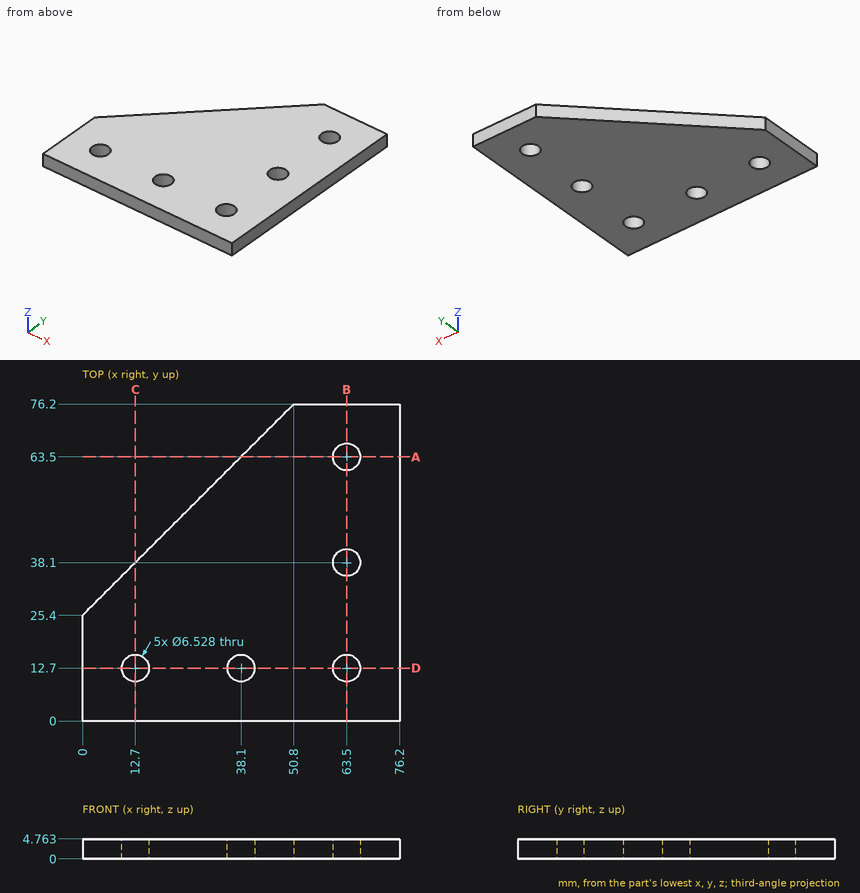
Job drawing, mm, ordinate dimensions from the low corner. One solid piece. Give positions to 0.01 mm unless a question says otherwise; leave off trailing zeros. Write each loop counter-clockwise with the first axis right and the second up, starting at its lowest first coordinate (ties: lowest second). Pieces come first, ordered by that corner, then holes. Notation, with made-up numbers: (89.5, 71.25) - (121.5, 71.25) arc R24 cw to (121.5, 103.25) - close; hole circle Ø5 at (28.25, -1.75). An arc over 180 degrees is marked (long way). Use one line per item in the form item = value. Start each with the question number.
1. Drop flat-ended pins along their axis: pin 1 Ø4 at (x, y) = (38.1, 12.7) entering from +Z; pin 2 Ø1 at (x, z) = (17, 2) entering from +Y. Give the stop position or say it passes through.
2. Band-saw the part on B-B on x = 63.5. Write the cut outline in (y, z).
3. Probe line 1 (Y direction, x = 63.5, z = 2.55); line 2 (X direction, y = 11.5, z = 3.35) (1 decimal); line 3 (Y direction, x = 65, z = 2.4). List the from-to ranges inside material, lowest first. Write a range as [from, to].
4. Band-saw the part on C-C on x = 12.7. Write the cut outline in (y, z).
5. Band-saw the part on A-A on y = 63.5. Write the cut outline in (x, z).
Conclusion:
q1.pin_1 = through
q1.pin_2 = 42.9
q2.outline = (0, 0) - (9.44, 0) - (9.44, 4.76) - (0, 4.76) - close; (15.96, 0) - (34.84, 0) - (34.84, 4.76) - (15.96, 4.76) - close; (41.36, 0) - (60.24, 0) - (60.24, 4.76) - (41.36, 4.76) - close; (66.76, 0) - (76.2, 0) - (76.2, 4.76) - (66.76, 4.76) - close
q3.line_1 = [0, 9.44], [15.96, 34.84], [41.36, 60.24], [66.76, 76.2]
q3.line_2 = [0, 9.7], [15.7, 35.1], [41.1, 60.5], [66.5, 76.2]
q3.line_3 = [0, 9.8], [15.6, 35.2], [41, 60.6], [66.4, 76.2]
q4.outline = (0, 0) - (9.44, 0) - (9.44, 4.76) - (0, 4.76) - close; (15.96, 0) - (38.1, 0) - (38.1, 4.76) - (15.96, 4.76) - close
q5.outline = (38.1, 0) - (60.24, 0) - (60.24, 4.76) - (38.1, 4.76) - close; (66.76, 0) - (76.2, 0) - (76.2, 4.76) - (66.76, 4.76) - close
